The drawing under review shows one solid part. Ordinate dimensions are in mm from its lowest x, y, z. Round coordinates to 2 decimals unless told otherwise and drop trailing zeros. Order: outer loops, then holes, each group sorted by start corner. A loop starts at its lowest first (then second) coordinate and runs counter-clockwise, first axis right, second up. Notation, with made-up numbers: M 82,31 L 112,31 A23 ccw 112,65 Z; hole C 86.5,70.5 d4. An arc over 180 degrees is marked long. Answer as a JSON object with one key per item and string values. Group by question number.
1. Add section C-C on y = 11.25. State the section outline as (x, z) points, and give its area (3 significant figures).
2. Add section B-B on x = 35. State the section outline as (y, z) points.
3. To check wall thickness, follow probe 1 along Z at (x, y) = (35, 7); probe 2 along X at (y, z) = (18.25, 31.5); probe 3 along X at (y, z) = (19.25, 26). State the ranges of each line that lie inside material, in increasing order. Write a range as [from, to].
4. Mouldability with a two-part tool opening along X and no side actions: class the marked faces 1, 2, 3 and 4 as released by +X, released by -X, zero draft, split by the parting line, or undercut.
5. Add section A-A on z = 47. State the section outline as (x, y) points.
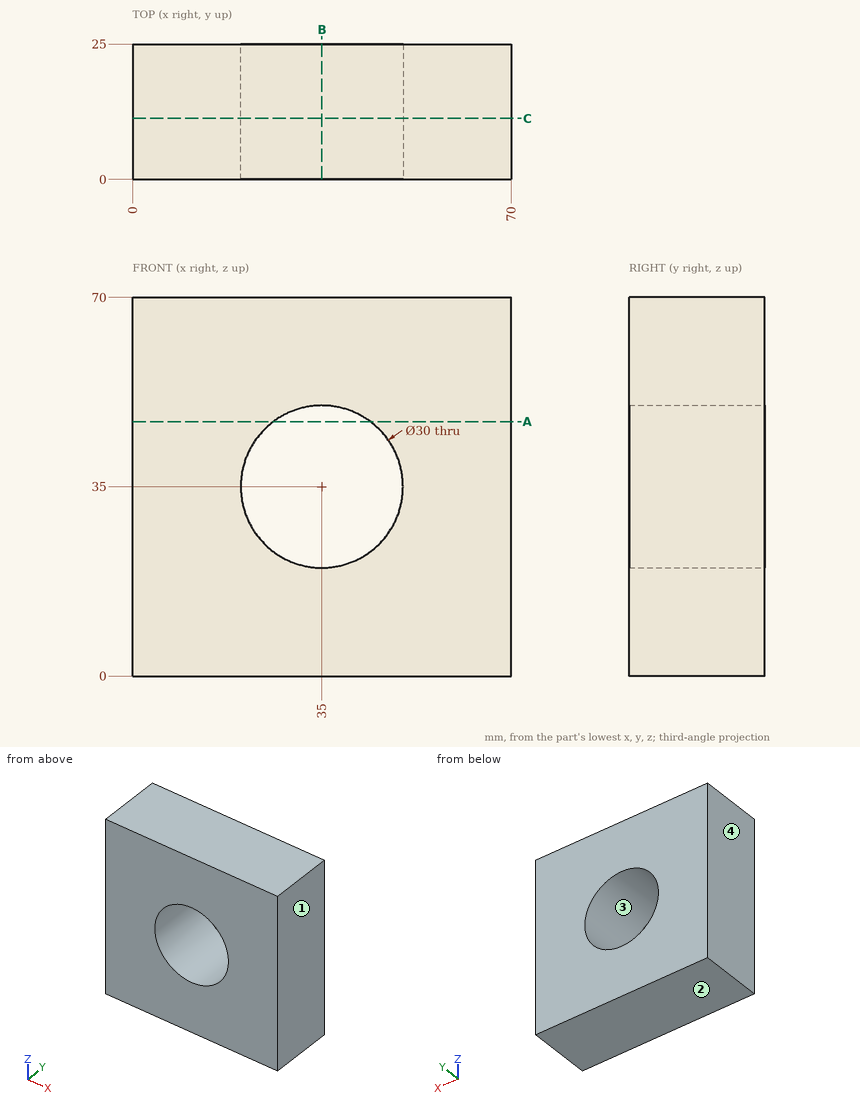
Recorded:
{
 "1": {"outline": "M 0,0 L 70,0 L 70,70 L 0,70 Z; hole C 35,35 d30", "area": "4,190 mm²"},
 "2": {"outline": "M 0,0 L 25,0 L 25,20 L 0,20 Z; M 0,50 L 25,50 L 25,70 L 0,70 Z"},
 "3": {"probe 1": "z = [0, 20], [50, 70]", "probe 2": "x = [0, 20.41], [49.59, 70]", "probe 3": "x = [0, 23], [47, 70]"},
 "4": {"face 1": "released by +X", "face 2": "zero draft", "face 3": "undercut", "face 4": "released by -X"},
 "5": {"outline": "M 0,0 L 26,0 L 26,25 L 0,25 Z; M 44,0 L 70,0 L 70,25 L 44,25 Z"}
}
